```python
from build123d import *

# Parameters (mm, degrees)
SKETCH1_R           = 10.75
BOSS_EXTRUDE1_DEPTH = 4
SKETCH2_R           = 4
CUT_EXTRUDE1_DEPTH  = 10
SKETCH3_R           = 20
SKETCH3_R_2         = 10.75
BOSS_EXTRUDE2_DEPTH = 19
SKETCH4_R           = 2
CUT_EXTRUDE2_DEPTH  = 20


with BuildPart() as part:
    # Sketch1 → Boss-Extrude1 (new body)
    with BuildSketch(Plane.XY):
        with BuildLine():
            Line((-70, -20), (70, -20))
            ThreePointArc((70, -20), (84.142136, -14.142136), (90, 0))
            Line((90, 0), (90, 88.85))
            Line((90, 88.85), (-89.389486, 88.85))
            Line((-89.389486, 88.85), (-90, 0))
            ThreePointArc((-90, 0), (-84.142136, -14.142136), (-70, -20))
        make_face()
        with Locations((70, 0)):
            Circle(SKETCH1_R, mode=Mode.SUBTRACT)
        with Locations((-70, 0)):
            Circle(SKETCH1_R, mode=Mode.SUBTRACT)
    extrude(amount=BOSS_EXTRUDE1_DEPTH)

    # Sketch2 → Cut-Extrude1 (cut)
    with BuildSketch(Plane.XY):
        with Locations((0.554741, 69)):
            Circle(SKETCH2_R)
    extrude(amount=CUT_EXTRUDE1_DEPTH, mode=Mode.SUBTRACT)

    # Sketch3 → Boss-Extrude2 (add)
    with BuildSketch(Plane.XY):
        with Locations((-70, 0)):
            Circle(SKETCH3_R)
        with Locations((-70, 0)):
            Circle(SKETCH3_R_2, mode=Mode.SUBTRACT)
        with Locations((70, 0)):
            Circle(SKETCH3_R)
        with Locations((70, 0)):
            Circle(SKETCH3_R_2, mode=Mode.SUBTRACT)
    extrude(amount=BOSS_EXTRUDE2_DEPTH)

    # Sketch4 → Cut-Extrude2 (cut)
    with BuildSketch(Plane(origin=(0, 0, 0), x_dir=(1, 0, 0), z_dir=(0, 1, 0))):
        with Locations((-70, -9.5)):
            Circle(SKETCH4_R)
        with Locations((70, -9.5)):
            Circle(SKETCH4_R)
    extrude(amount=-CUT_EXTRUDE2_DEPTH, mode=Mode.SUBTRACT)


solid = part.part
```
Geometry: final body of the model. Coordinates: model frame, mm. A direction names the side the tool comes from. Round coordinates to 2 decimals unless told otherwise and drop trailing zeros. Write each loop counter-clockwise with the first axis right and the second up, starting at its lowest first coordinate (ties: lowest second). Pieces come first, ordered by that corner, then holes. Notation, with made-up numbers: M 19.25,-11.5 L 36.25,-11.5 A18 ccw 36.25,-1.5 Z; hole C 37,-18 d11. An arc over 180 degrees is marked long. Answer in a Markdown table with one row per item. Add a question column.
(1) Ray query, L1, parallel to X at y = 4, z = 1.5; L2, parallel to X at y = 5, z = 11; L3, parallel to X at y = -15, z = 9.5. Return the intervals inside material, ascending.
(2) Contact query for flat-ended pins moving along their axis: pin 1 (10 mm diameter, centred on x = 53, z = 10.5, fed in from +Y); pin 2 (3 mm diameter, centred on x = -3.5, y = -1, fed in from +Z); pin 3 (5 mm diameter, centred on x = 70, z = 9.5, fed in from +Y). Output: stop coordinate, or through.
(3) Cut plane D-D, the plane x = 62.5. Return the cut outline in (y, z), then the cut area to 3 significant figures.
(4) Cut plane B-B, the plane y = 69. Return the cut outline in (x, z).
(5) Cut plane A-A, the plane z = 17.25. Return the cut outline in (x, y).
(6) Reachability of faces 5 (the face through (-68.092, -15.213, 8.899)), 6 (the face through (-59.746, 3.229, 9.367)) from +Z, -Z, +X, -X, +Y, -Y: full face, straight path, thin tool, end or side. Return the list, or none.
(7) Draft query along Z for faces 1 (the face through (71.908, -15.213, 8.899)), 2 (the face through (79, -9, 19)), 3 (the face through (-0.312, 65.095, 1.972)), 4 (the face through (-1, 35, 0)). Return one class per face: pulls with the +Z half, pulls with the -Z half, needs draft (parallel to the pull), parting line crosses it, or undercut.
(8) Cut plane C-C, the plane z = 9.5. Return the cut outline in (x, y).
Established:
| question | item | result |
|---|---|---|
| 1 | L1 | -89.97 to -79.98, -60.02 to 60.02, 79.98 to 90 |
| 1 | L2 | -89.36 to -79.52, -60.48 to -50.64, 50.64 to 60.48, 79.52 to 89.36 |
| 1 | L3 | -83.23 to -72, -68 to -56.77, 56.77 to 68, 72 to 83.23 |
| 2 | pin 1 | y = 16 |
| 2 | pin 2 | z = 4 |
| 2 | pin 3 | y = 20 |
| 3 | outline | M -20,0 L -7.7,0 L -7.7,19 L -18.54,19 L -18.54,4 L -20,4 Z; M 7.7,0 L 88.85,0 L 88.85,4 L 18.54,4 L 18.54,19 L 7.7,19 Z |
| 3 | area | 699 mm² |
| 4 | outline | M -89.53,0 L -3.45,0 L -3.45,4 L -89.53,4 Z; M 4.55,0 L 90,0 L 90,4 L 4.55,4 Z |
| 5 | outline | C -70,0 d40; C 70,0 d40; hole C -70,0 d21.5; hole C 70,0 d21.5 |
| 6 | face 5 | -Y |
| 6 | face 6 | +Z, -Z |
| 7 | face 1 | undercut |
| 7 | face 2 | pulls with the +Z half |
| 7 | face 3 | needs draft |
| 7 | face 4 | pulls with the -Z half |
| 8 | outline | M -72,-19.9 L -72,-10.56 A10.75 cw long -68,-10.56 L -68,-19.9 A20 ccw long Z; M 68,-19.9 L 68,-10.56 A10.75 cw long 72,-10.56 L 72,-19.9 A20 ccw long Z |
